Read the model definition and answer for the solid it produces. Units are mm, in the model's axes. A direction names the side the tool comes from. Coordinates: 2 decimals unless noted, no trailing zeros. Loops run counter-clockwise (first coordinate to the right, second up) from the corner with the lowest first, then second, coordinate; pieces in that order, holes last.
Autodesk Inventor part; units mm, degrees
ref_plane "YZ Plane" through (0, 0, 0) normal (1, 0, 0) x (0, 1, 0)
ref_plane "XZ Plane" through (0, 0, 0) normal (0, 1, 0) x (-1, 0, 0)
ref_plane "XY Plane" through (0, 0, 0) normal (0, 0, 1) x (1, 0, 0)
sketch "Sketch1" plane through (0, 0, 0) normal (0, 1, 0) x (-1, 0, 0)
  line L0 (0, 0) -> (-77.789, 0) construction
  line L1 (0, 4) -> (-77.789, 4)
  line L2 (-77.789, -4) -> (0, -4)
  arc A0 (0, -4) -> (0, 4) centre (0, 0) ccw
  arc A1 (-77.789, 4) -> (-77.789, -4) centre (-77.789, 0) ccw
  circle A2 centre (0, 0) radius 2.1
  circle A3 centre (-77.789, 0) radius 2.1
  point P0 (-38.8945, 0)
  dimension "d0" = 77.789
  dimension "d1" = 8
  dimension "d2" = 4.2
  dimension "d10" = 4.2
extrude "Extrusion1" add sketch "Sketch1" along normal blind 5
sketch "Sketch2" plane through (0, 5, 0) normal (0, 1, 0) x (1, 0, 0)
  arc A0 (77.789, -4) -> (77.789, 4) centre (77.789, 0) ccw
  line L0 (77.789, 4) -> (0, 4)
  arc A1 (0, 4) -> (0, -4) centre (0, 0) ccw
  line L1 (0, -4) -> (77.789, -4)
  circle A2 centre (77.789, 0) radius 2.1
  circle A3 centre (0, 0) radius 2.1
  circle A4 centre (8, 0) radius 4
  line L2 (0, -4) -> (77.789, -4)
  circle A5 centre (69.789, 0) radius 4
  point P0 (69.789, -4)
  point P1 (69.789, 4)
  point P2 (8, -4)
  point P3 (8, 4)
  dimension "d11" = 8
  dimension "d12" = 8
  dimension "d13" = 8
extrude "Extrusion2" add sketch "Sketch2" along normal blind 10 contours L1 A1 L0 A4 | A4
Item 1: Which of the six approach directions +Z, -Z, +X, -X, +Y, -Y give full straight-line access (tool end or side, diameter ignored) to faces 4 (the face through (31, 4, -4)), 5 (the face through (12, 10, 0))?
Numbers:
face 4: -Z, +X, -X, +Y, -Y
face 5: +X, +Y
Item 2: Given pin 1 (4 mm diameter, centred on x = 49, z = 0.5, fed in from +Y); pin 2 (2.5 mm diameter, centred on x = 0, z = 0, fed in from +Y), each flat-ended and moving along its own axis, determine where each tip first touches the part or whether it passes through.
Numbers:
pin 1: stops at y = 5
pin 2: passes through
Item 3: Find the intervals of material crossed by line 1 along X through (y, z) = (2.75, -1.5); line 2 along Y through (x, z) = (65.5, 2); line 3 along Z through (x, y) = (0, 7.75), in increasing order.
Numbers:
line 1: x = -3.71 to -1.47, 1.47 to 76.32, 79.26 to 81.5
line 2: y = 0 to 5
line 3: z = -4 to -2.1, 2.1 to 4
Item 4: A cutting plane is placed at C-C on x = 33.5. Determine the outline of the cut face in (y, z), then the cut area to 3 significant figures.
Numbers:
outline: (0, -4) - (5, -4) - (5, 4) - (0, 4) - close
area: 40.0 mm2
Item 5: A cutting plane is placed at B-B on y = 5.75. Determine the outline of the cut face in (x, z), then the cut area to 3 significant figures.
Numbers:
outline: (0, -4) - (8, -4) arc R4 ccw to (8, 4) - (0, 4) arc R4 ccw to start; hole circle Ø4.2 at (0, 0)
area: 100 mm2
Item 6: Determine the mould class of faces 1 (the face through (79.887, 2.465, -0.092)), 2 (the face through (-4, 7, 0)), 3 (the face through (39, 0, 0)) for opening direction X: released by +X, released by -X, zero draft, split by the parting line, or undercut.
Numbers:
face 1: undercut
face 2: released by -X
face 3: zero draft
Item 7: A cutting plane is placed at D-D on x = 9.5. Determine the outline of the cut face in (y, z), then the cut area to 3 significant figures.
Numbers:
outline: (0, -4) - (5, -4) - (5, -3.71) - (15, -3.71) - (15, 3.71) - (5, 3.71) - (5, 4) - (0, 4) - close
area: 114 mm2
Item 8: A cutting plane is placed at A-A on y = 2.5. Determine the outline of the cut face in (x, z), then the cut area to 3 significant figures.
Numbers:
outline: (0, -4) - (77.79, -4) arc R4 ccw to (77.79, 4) - (0, 4) arc R4 ccw to start; hole circle Ø4.2 at (0, 0); hole circle Ø4.2 at (77.79, 0)
area: 645 mm2
